Input: part model. Units: mm. Frame: model coordinates. Coordinates: 2 decimals unless noted, no trailing zeros. Order: outer loops, then holes, each group sorted by start corner. A loop starts at its lowest first (then second) coordinate and runs counter-clockwise, first axis right, second up. Notation, with made-up numbers: (74, 15.25) -> (124, 15.25) arc R18 ccw to (124, 43.25) -> close; hole circle Ø5 at (38, 64). An arc over 180 degrees is marked (long way). One line per item, written item: value. Start each with the question number.
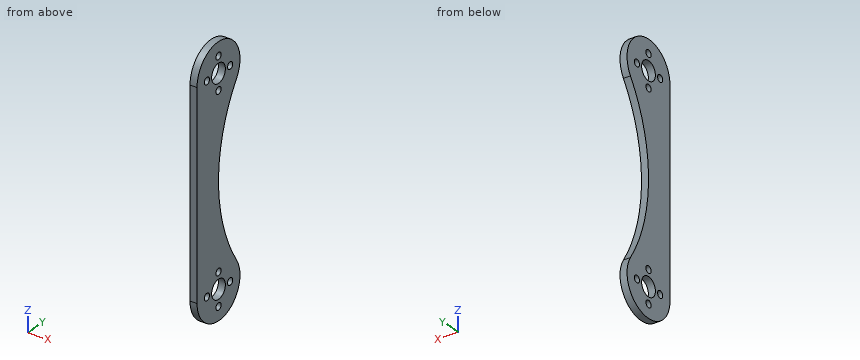
from build123d import *

# Parameters (mm, degrees)
SKETCH1_R           = 4
SKETCH1_R_2         = 1.5
BOSS_EXTRUDE1_DEPTH = 3


with BuildPart() as part:
    # Sketch1 → Boss-Extrude1 (new body)
    with BuildSketch(Plane(origin=(0, 0, 0), x_dir=(0, 0, -1), z_dir=(1, 0, 0))):
        with BuildLine():
            Line((-42.55, -12.5), (42.55, -12.5))
            ThreePointArc((42.55, -12.5), (54.543190221, 3.523263872), (35.789172189, 10.51385787))
            ThreePointArc((35.789172189, 10.51385787), (0, 0), (-35.789172189, 10.51385787))
            ThreePointArc((-35.789172189, 10.51385787), (-54.543190221, 3.523263872), (-42.55, -12.5))
        make_face()
        with Locations((-42.55, 0)):
            Circle(SKETCH1_R, mode=Mode.SUBTRACT)
        with Locations((-35.775, 0)):
            Circle(SKETCH1_R_2, mode=Mode.SUBTRACT)
        with Locations((-42.55, -6.775)):
            Circle(SKETCH1_R_2, mode=Mode.SUBTRACT)
        with Locations((-49.325, 0)):
            Circle(SKETCH1_R_2, mode=Mode.SUBTRACT)
        with Locations((-42.55, 6.775)):
            Circle(SKETCH1_R_2, mode=Mode.SUBTRACT)
        with Locations(Location((42.55, 6.775, 0), (0, 0, 180))):
            Circle(SKETCH1_R_2, mode=Mode.SUBTRACT)
        with Locations(Location((49.325, 0, 0), (0, 0, 180))):
            Circle(SKETCH1_R_2, mode=Mode.SUBTRACT)
        with Locations(Location((42.55, -6.775, 0), (0, 0, 180))):
            Circle(SKETCH1_R_2, mode=Mode.SUBTRACT)
        with Locations(Location((35.775, 0, 0), (0, 0, 180))):
            Circle(SKETCH1_R_2, mode=Mode.SUBTRACT)
        with Locations(Location((42.55, 0, 0), (0, 0, 180))):
            Circle(SKETCH1_R, mode=Mode.SUBTRACT)
    extrude(amount=BOSS_EXTRUDE1_DEPTH)


solid = part.part
1) Section query B-B, the plane x = 1.4. State how many separate pieces and enclosed holes the cut face has, plus the area to 3 significant figures.
2) Section query A-A, the plane z = -40. Return the cut outline in (x, y).
3) Ray query, line 1 along Y through (x, z) = (1.95, 42.55) (3 decimals); line 2 along Z through (x, y) = (1.9, 5.5); line 3 along Z through (x, y) = (0.6, 7). Return the intervals inside material, ascending. Write a range as from..to.
4) Pin query (flat end, axial travel): pin 1 Ø1.8 at (y, z) = (0, 35.775) entering from -X; pin 2 Ø1 at (x, y) = (2, 8.5) entering from +Z. Return the tip coordinate at first contact, or that it passes through.
Entries:
1. separate pieces: 1
1. enclosed holes: 10
1. area: 1,800 mm2
2. outline: (0, -12.5) -> (3, -12.5) -> (3, -3.08) -> (0, -3.08) -> close; (0, 3.08) -> (3, 3.08) -> (3, 12.24) -> (0, 12.24) -> close
3. line 1: y = -12.5..-8.275, -5.275..-4, 4..5.275, 8.275..12.5
3. line 2: z = -53.77..-43.34, -41.76..-26.41, 26.41..41.76, 43.34..53.77
3. line 3: z = -52.91..-44.03, -41.07..-29.62, 29.62..41.07, 44.03..52.91
4. pin 1: passes through
4. pin 2: stops at z = 52.15
